Work out the finished part from the listing and answer in its coordinate system (mm). A direction names the side the tool comes from. Coordinates: 2 decimals unless noted, no trailing zeros. Order: outer loops, then holes, each group sorted by start corner. A loop starts at its lowest first (then second) coordinate and runs counter-clockwise, first axis right, second up. Notation, with made-up numbers: (44.5, -32) -> (92.5, -32) arc R20 ccw to (92.5, -9) -> close; hole circle Ø7 at (46, 2). An arc over 180 degrees is marked (long way). Write item = value, one per line. Start each with the question number.
Q1. Straight lines are drawn through the part: L1, parallel to X at y = 6.5, z = 2.5; L2, parallel to Y at x = 60, z = 9.5. For each, find the intervals that lie inside material, in ascending order. Write a range as from..to.
Q2. The part is cut by section D-D, the plane z = -18. Determine the outline of the cut face in (x, y).
Q3. The part is cut by section C-C, the plane y = 34.5. Determine the outline of the cut face in (x, z).
Q4. The part is cut by section A-A, the plane z = 0. Determine the outline of the cut face in (x, y), plus the area to 3 significant figures.
Q5. For a pull along X with two mould halves and no side action, classify faces 4 (the cylindrical face through (45.9, -1.5, 18)), 5 (the flat face through (0, -2, 0)), 6 (the cylindrical face through (68.52, 53.39, -21.58)) as +X half, -X half, draft (parallel to the pull), parting line (faces both ways), or undercut.
Q6. Which of the six approach directions +Z, -Z, +X, -X, +Y, -Y give full straight-line access (tool end or side, diameter ignored) to faces 1 (the flat face through (15, -1, -15.9)), 2 (the flat face through (67, 15, 0)), 3 (the cylindrical face through (68.479, 22.724, -12.467))?
Q7. The part is cut by section B-B, the plane x = 14. Determine the outline of the cut face in (y, z).
Q8. A flat-ended cylindrical pin translates along its axis: pin 1 (3 mm diameter, centred on x = 51, z = -16.5, fed in from +Y). Find the tip coordinate at first contact, or state that the pin passes through.
```python
from build123d import *

# Parameters (mm, degrees)
EXTRUDE_1_DEPTH     = 25
CUT_EXTRUDE_1_REACH = 95.67
CUT_EXTRUDE_2_REACH = 95.67
SKETCH_3_R          = 13.1
SKETCH_3_R_2        = 2.1
FILLET_1_R          = 12


with BuildPart() as part:
    # 草图1 → 凸台-拉伸1 (new, symmetric)
    with BuildSketch(Plane.XY):
        Polygon((0, 0), (67, 0), (67, 57), (70, 57), (70, -3), (0, -3), align=None)
    extrude(amount=EXTRUDE_1_DEPTH, both=True)

    # 草图2 → 切除-拉伸1 (cut, up to next)
    with BuildSketch(Plane(origin=(0, 0, 0), x_dir=(1, 0, 0), z_dir=(0, 1, 0)), mode=Mode.PRIVATE) as cut_extrude_1_sk1:
        with BuildLine():
            Line((11, 20.1), (19, 20.1))
            ThreePointArc((19, 20.1), (21.1, 18), (19, 15.9))
            Line((19, 15.9), (11, 15.9))
            ThreePointArc((11, 15.9), (8.9, 18), (11, 20.1))
        make_face()
    cut_extrude_1_tool1 = extrude(cut_extrude_1_sk1.sketch, amount=-CUT_EXTRUDE_1_REACH, mode=Mode.PRIVATE) & part.part
    # 草图2 → 切除-拉伸1 (cut, up to next)
    with BuildSketch(Plane(origin=(0, 0, 0), x_dir=(1, 0, 0), z_dir=(0, 1, 0)), mode=Mode.PRIVATE) as cut_extrude_1_sk2:
        with BuildLine():
            Line((48, 20.1), (56, 20.1))
            ThreePointArc((56, 20.1), (58.1, 18), (56, 15.9))
            Line((56, 15.9), (48, 15.9))
            ThreePointArc((48, 15.9), (45.9, 18), (48, 20.1))
        make_face()
    cut_extrude_1_tool2 = extrude(cut_extrude_1_sk2.sketch, amount=-CUT_EXTRUDE_1_REACH, mode=Mode.PRIVATE) & part.part
    # 草图2 → 切除-拉伸1 (cut, up to next)
    with BuildSketch(Plane(origin=(0, 0, 0), x_dir=(1, 0, 0), z_dir=(0, 1, 0)), mode=Mode.PRIVATE) as cut_extrude_1_sk3:
        with BuildLine():
            Line((11, -20.1), (19, -20.1))
            ThreePointArc((19, -20.1), (21.1, -18), (19, -15.9))
            Line((19, -15.9), (11, -15.9))
            ThreePointArc((11, -15.9), (8.9, -18), (11, -20.1))
        make_face()
    cut_extrude_1_tool3 = extrude(cut_extrude_1_sk3.sketch, amount=-CUT_EXTRUDE_1_REACH, mode=Mode.PRIVATE) & part.part
    # 草图2 → 切除-拉伸1 (cut, up to next)
    with BuildSketch(Plane(origin=(0, 0, 0), x_dir=(1, 0, 0), z_dir=(0, 1, 0)), mode=Mode.PRIVATE) as cut_extrude_1_sk4:
        with BuildLine():
            Line((48, -20.1), (56, -20.1))
            ThreePointArc((56, -20.1), (58.1, -18), (56, -15.9))
            Line((56, -15.9), (48, -15.9))
            ThreePointArc((48, -15.9), (45.9, -18), (48, -20.1))
        make_face()
    cut_extrude_1_tool4 = extrude(cut_extrude_1_sk4.sketch, amount=-CUT_EXTRUDE_1_REACH, mode=Mode.PRIVATE) & part.part
    add(cut_extrude_1_tool1.solids().sort_by_distance((15, 0, -18))[0], mode=Mode.SUBTRACT)
    add(cut_extrude_1_tool2.solids().sort_by_distance((52, 0, -18))[0], mode=Mode.SUBTRACT)
    add(cut_extrude_1_tool3.solids().sort_by_distance((15, 0, 18))[0], mode=Mode.SUBTRACT)
    add(cut_extrude_1_tool4.solids().sort_by_distance((52, 0, 18))[0], mode=Mode.SUBTRACT)

    # 草图3 → 切除-拉伸2 (cut, up to next)
    with BuildSketch(Plane(origin=(0, 0, 0), x_dir=(0, 0, -1), z_dir=(1, 0, 0)), mode=Mode.PRIVATE) as cut_extrude_2_sk1:
        with Locations(Location((0, 33, 0), (0, 0, 270))):
            Circle(SKETCH_3_R)
    cut_extrude_2_tool1 = extrude(cut_extrude_2_sk1.sketch, amount=CUT_EXTRUDE_2_REACH, mode=Mode.PRIVATE) & part.part
    # 草图3 → 切除-拉伸2 (cut, up to next)
    with BuildSketch(Plane(origin=(0, 0, 0), x_dir=(0, 0, -1), z_dir=(1, 0, 0)), mode=Mode.PRIVATE) as cut_extrude_2_sk2:
        with Locations(Location((12.374368671, 45.374368671, 0), (0, 0, 270))):
            Circle(SKETCH_3_R_2)
    cut_extrude_2_tool2 = extrude(cut_extrude_2_sk2.sketch, amount=CUT_EXTRUDE_2_REACH, mode=Mode.PRIVATE) & part.part
    # 草图3 → 切除-拉伸2 (cut, up to next)
    with BuildSketch(Plane(origin=(0, 0, 0), x_dir=(0, 0, -1), z_dir=(1, 0, 0)), mode=Mode.PRIVATE) as cut_extrude_2_sk3:
        with Locations(Location((12.374368671, 20.625631329, 0), (0, 0, 270))):
            Circle(SKETCH_3_R_2)
    cut_extrude_2_tool3 = extrude(cut_extrude_2_sk3.sketch, amount=CUT_EXTRUDE_2_REACH, mode=Mode.PRIVATE) & part.part
    # 草图3 → 切除-拉伸2 (cut, up to next)
    with BuildSketch(Plane(origin=(0, 0, 0), x_dir=(0, 0, -1), z_dir=(1, 0, 0)), mode=Mode.PRIVATE) as cut_extrude_2_sk4:
        with Locations(Location((-12.374368671, 20.625631329, 0), (0, 0, 270))):
            Circle(SKETCH_3_R_2)
    cut_extrude_2_tool4 = extrude(cut_extrude_2_sk4.sketch, amount=CUT_EXTRUDE_2_REACH, mode=Mode.PRIVATE) & part.part
    # 草图3 → 切除-拉伸2 (cut, up to next)
    with BuildSketch(Plane(origin=(0, 0, 0), x_dir=(0, 0, -1), z_dir=(1, 0, 0)), mode=Mode.PRIVATE) as cut_extrude_2_sk5:
        with Locations(Location((-12.374368671, 45.374368671, 0), (0, 0, 270))):
            Circle(SKETCH_3_R_2)
    cut_extrude_2_tool5 = extrude(cut_extrude_2_sk5.sketch, amount=CUT_EXTRUDE_2_REACH, mode=Mode.PRIVATE) & part.part
    add(cut_extrude_2_tool1.solids().sort_by_distance((0, 33, 0))[0], mode=Mode.SUBTRACT)
    add(cut_extrude_2_tool2.solids().sort_by_distance((0, 45.374369, -12.374369))[0], mode=Mode.SUBTRACT)
    add(cut_extrude_2_tool3.solids().sort_by_distance((0, 20.625631, -12.374369))[0], mode=Mode.SUBTRACT)
    add(cut_extrude_2_tool4.solids().sort_by_distance((0, 20.625631, 12.374369))[0], mode=Mode.SUBTRACT)
    add(cut_extrude_2_tool5.solids().sort_by_distance((0, 45.374369, 12.374369))[0], mode=Mode.SUBTRACT)

    # 圆角1
    fillet_1_edges = [part.edges().sort_by_distance(p)[0] for p in [
        (68.5, 57, 25),
        (68.5, 57, -25),
    ]]
    fillet(fillet_1_edges, radius=FILLET_1_R)


solid = part.part
```
Model answer:
q1.L1 = 67..70
q1.L2 = -3..0
q2.outline = (0, -3) -> (8.9, -3) -> (8.9, 0) -> (0, 0) -> close; (21.1, -3) -> (45.9, -3) -> (45.9, 0) -> (21.1, 0) -> close; (58.1, -3) -> (70, -3) -> (70, 55.91) -> (67, 55.91) -> (67, 0) -> (58.1, 0) -> close
q3.outline = (67, -25) -> (70, -25) -> (70, -13.01) -> (67, -13.01) -> close; (67, 13.01) -> (70, 13.01) -> (70, 25) -> (67, 25) -> close
q4.outline = (0, -3) -> (70, -3) -> (70, 19.9) -> (67, 19.9) -> (67, 0) -> (0, 0) -> close; (67, 46.1) -> (70, 46.1) -> (70, 57) -> (67, 57) -> close
q4.area = 302 mm2
q5.face_4 = undercut
q5.face_5 = -X half
q5.face_6 = draft
q6.face_1 = +Y, -Y
q6.face_2 = +Z, -Z, -X, +Y
q6.face_3 = +X, -X
q7.outline = (-3, -25) -> (0, -25) -> (0, -20.1) -> (-3, -20.1) -> close; (-3, -15.9) -> (0, -15.9) -> (0, 15.9) -> (-3, 15.9) -> close; (-3, 20.1) -> (0, 20.1) -> (0, 25) -> (-3, 25) -> close
q8.pin_1 = 0
